```python
from build123d import *

# Parameters (mm, degrees)
EXTRUDE_DEPTH   = 30
POCKET_DEPTH    = 22.001
POCKET001_DEPTH = 7
POCKET002_DEPTH = 3
POCKET003_DEPTH = 3
SKETCH005_R     = 4.05
POCKET004_DEPTH = 18


with BuildPart() as part:
    # Sketch → Extrude (new body)
    with BuildSketch(Plane.XY):
        with BuildLine():
            ThreePointArc((-5.852556, 1.533), (-6.046854, -0.195073), (-5.741579, -1.907031))
            Line((-5.741579, -1.907031), (-4.05, -7))
            Line((-4.05, -7), (4.05, -7))
            Line((4.05, -7), (5.741579, -1.907031))
            ThreePointArc((5.741579, -1.907031), (6.046854, -0.195073), (5.852556, 1.533))
            Line((2.325, 15), (5.852556, 1.533))
            Line((0.325, 15), (2.325, 15))
            Line((0.325, 0.945714), (0.325, 15))
            ThreePointArc((-0.325, 0.945714), (0, -1), (0.325, 0.945714))
            Line((-0.325, 15), (-0.325, 0.945714))
            Line((-2.325, 15), (-0.325, 15))
            Line((-5.852556, 1.533), (-2.325, 15))
        make_face()
    extrude(amount=EXTRUDE_DEPTH)

    # Sketch001 → Pocket (cut, through all)
    with BuildSketch(Plane.XZ.offset(7)):
        with BuildLine():
            Line((-6.05, 30), (0, 30))
            Line((0, 30), (6.05, 30))
            ThreePointArc((-6.05, 30), (0, 28.641403), (6.05, 30))
        make_face()
    extrude(amount=-POCKET_DEPTH, mode=Mode.SUBTRACT)

    # Sketch002 → Pocket001 (cut)
    with BuildSketch(Plane.XZ.offset(7)):
        with BuildLine():
            Line((-4.05, 29.23338), (-4.05, 26.23338))
            Line((-4.05, 26.23338), (4.05, 26.23338))
            Line((4.05, 26.23338), (4.05, 29.23338))
            ThreePointArc((-4.05, 29.23338), (0, 28.641403), (4.05, 29.23338))
        make_face()
    extrude(amount=-POCKET001_DEPTH, mode=Mode.SUBTRACT)

    # Sketch003 → Pocket002 (cut)
    with BuildSketch(Plane.XY.offset(26.23338)):
        with BuildLine():
            ThreePointArc((1.55, -3.5), (0, -1.95), (-1.55, -3.5))
            Line((-1.55, -3.5), (-1.55, -7))
            Line((-1.55, -7), (1.55, -7))
            Line((1.55, -7), (1.55, -3.5))
        make_face()
    extrude(amount=-POCKET002_DEPTH, mode=Mode.SUBTRACT)

    # Sketch004 → Pocket003 (cut)
    with BuildSketch(Plane.XY.offset(23.23338)):
        with BuildLine():
            ThreePointArc((3.05, -3.5), (0, -0.45), (-3.05, -3.5))
            Line((-3.05, -3.5), (-3.05, -7))
            Line((-3.05, -7), (3.05, -7))
            Line((3.05, -7), (3.05, -3.5))
        make_face()
    extrude(amount=-POCKET003_DEPTH, mode=Mode.SUBTRACT)

    # Sketch005 → Pocket004 (cut)
    with BuildSketch(Plane(origin=(0, 0, 0), x_dir=(1, 0, 0), z_dir=(0, 0, -1))):
        Circle(SKETCH005_R)
    extrude(amount=-POCKET004_DEPTH, mode=Mode.SUBTRACT)


solid = part.part
```
Build history of the part. All positions in model axes, mm. A direction names the side the tool comes from. Coordinates: 2 decimals unless noted, no trailing zeros. Order: outer loops, then holes, each group sorted by start corner. A loop starts at its lowest first (then second) coordinate and runs counter-clockwise, first axis right, second up. Notation, with made-up numbers: M 23.5,-11.75 L 40.5,-11.75 A27 ccw 40.5,14.25 Z; hole C 5.5,23.25 d8. An arc over 180 degrees is marked long. One line per question, with ' | ' between items. Start each with the question number.
1. Cut at D-D (x = 2). Write the cut outline in (y, z).
2. Tool access for faces 1 (the face through (3, 0, 27)), 2 (the face through (-2.7, 6.3, 28.9)), 3 (the face through (-1, -2, 23.233)): list every direction of +Z, -Z, +X, -X, +Y, -Y with a clear straight run to the whole face (end or side of a thin tool).
3. Cut at A-A (x = 0). Write the cut outline in (y, z).
4. Flat gauge pins, fed straight in: P1, Ø1.5, axis at y = 4, z = 12.5, coming from the +X side; P2, Ø1.8, axis at x = 1.5, y = -2.5, coming from the -Z side; P3, Ø1.5, axis at y = -3, z = 28.5, coming from the +X side. Where does each tip first touch, or does it go through?
5. Cut at B-B (z = 7). Write the cut outline in (x, y) (3 decimals), plus the area to 3 significant figures.
6. Cut at C-C (y = 2.75). Write the cut outline in (x, z) (3 decimals).
7. Mould opens along Y. For faces 4 (the face through (1, 15, 14)), 5 (the face through (-3, 0, 28)), 6 (the face through (0.325, 9, 14)), 7 (the face through (-0.6, 0.8, 23.3)) say: +Y half, -Y half, draft (parallel to the pull), parting line (faces both ways), or undercut.
8. Wall check: line 1 along X through (y, z) = (12.25, 8.5) (3 decimals); line 2 along X through (y, z) = (0, 25); line 3 along Z through (x, y) = (-2.25, -2.5). Give the ranges that are in metal, low to high. Write a range as [from, to].
The answers:
1) outline: M -7,0 L -3.52,0 L -3.52,18 L 3.52,18 L 3.52,0 L 15,0 L 15,28.78 L 0,28.78 L 0,26.23 L -7,26.23 L -7,23.23 L -1.2,23.23 L -1.2,20.23 L -7,20.23 Z
2) face 1: +Z, -Y | face 2: +Z, +Y, -Y | face 3: -Y
3) outline: M -7,0 L -4.05,0 L -4.05,18 L -1,18 L -1,20.23 L -7,20.23 Z; M -1.95,23.23 L -1,23.23 L -1,26.23 L -1.95,26.23 Z
4) P1: stops at x = 5.4 | P2: stops at z = 18 | P3: stops at x = 5.63
5) outline: M -5.853,1.533 A6.05 ccw -5.742,-1.907 L -4.05,-7 L 4.05,-7 L 5.742,-1.907 A6.05 ccw 5.853,1.533 L 2.325,15 L 0.325,15 L 0.325,4.037 A4.05 cw long -0.325,4.037 L -0.325,15 L -2.325,15 Z | area: 142 mm2
6) outline: M -5.534,0 L -2.973,0 L -2.973,18 L -0.325,18 L -0.325,28.645 A14.15 cw -5.534,29.768 Z; M 0.325,18 L 2.973,18 L 2.973,0 L 5.534,0 L 5.534,29.768 A14.15 cw 0.325,28.645 Z
7) face 4: +Y half | face 5: -Y half | face 6: draft | face 7: undercut
8) line 1: x = [-3.045, -0.325], [0.325, 3.045] | line 2: x = [-6.05, -1], [1, 6.05] | line 3: z = [18, 20.23], [23.23, 26.23]
